Could you check a few things on this model? Use its own coordinates, in mm. Face numbers are marked on the shaded views. A direction names the side the tool comes from. Give positions to 0.01 mm unless a question says otherwise; leave off trailing zeros. Write each loop counter-clockwise with the first axis right and the second up, starting at its lowest first coordinate (ties: lowest second). Pieces come first, ordered by that corner, then holes. Notation, with made-up numbers: M 7.25,59 L 47.25,59 A20 cw 47.25,95 Z; hole C -16.75,42 d11. An arc over 180 degrees is marked long. One line per item, written item: value.
```python
from build123d import *

# Parameters (mm, degrees)
F0_R     = 7.3
F1_DEPTH = 2
F2_R     = 5
F3_DEPTH = 2
F4_SIZE  = 0.5
F5_R     = 2
F6_DEPTH = 4.001


with BuildPart() as f1:
    # F0 (on Top) → F1 (new body)
    with BuildSketch(Plane.XY):
        Circle(F0_R)
    extrude(amount=F1_DEPTH)

    # F2 (on face) → F3 (join)
    with BuildSketch(Plane.XY.offset(2)):
        Circle(F2_R)
    extrude(amount=F3_DEPTH)

    # F4
    f4_edges = [f1.edges().sort_by_distance(p)[0] for p in [
        (-7.3, 0, 0),
    ]]
    chamfer(f4_edges, length=F4_SIZE)

    # F5 (on face) → F6 (cut, through all)
    with BuildSketch(Plane(origin=(0, 0, 0), x_dir=(1, 0, 0), z_dir=(0, 0, -1))):
        Circle(F5_R)
    extrude(amount=-F6_DEPTH, mode=Mode.SUBTRACT)


solid = f1.part
```
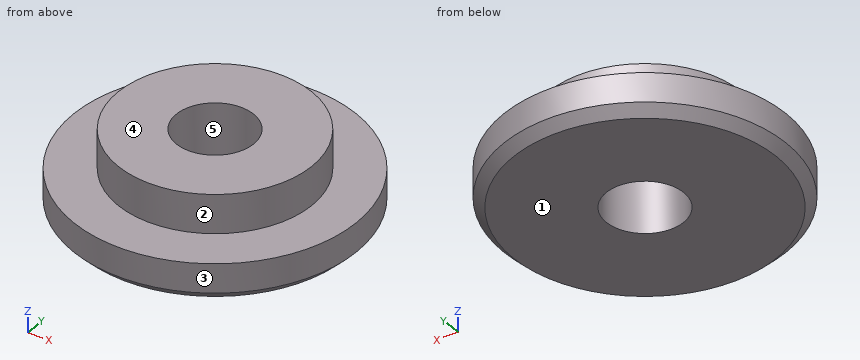
1) On a 3-axis mill with a long thin cutter (end or side, diameter ignored), from which of +Z, -Z, +X, -X, +Y, -Y can I reach the whole of each face in a straight line? I mean the marked faces 1 and 2. Say none if no direction works.
Outcome:
face 1: -Z, +X, -X, +Y, -Y
face 2: +Z
2) Please list where these lines run through material, in increasing order: L1, parallel to Y at x = 0, z = 0.95; L2, parallel to Y at x = 0, z = 2.85; L3, parallel to Z at x = 3.25, y = 5.25. Write a range as from..to.
Outcome:
L1: y = -7.3..-2, 2..7.3
L2: y = -5..-2, 2..5
L3: z = 0..2
3) If we section it at C-C, the plane z = 2.5: Write out the boundary of the cut face in (x, y).
Outcome:
outline: C 0,0 d10; hole C 0,0 d4
4) We'd pull the mould along Y, two halves only. Please class the marked faces 3, 4 and 5: pulls with the +Y half, pulls with the -Y half, needs draft (parallel to the pull), parting line crosses it, or undercut.
Outcome:
face 3: parting line crosses it
face 4: needs draft
face 5: undercut
5) If we section it at A-A, the plane y = 0: Write out the boundary of the cut face in (x, z), then the cut area to 4 significant figures.
Outcome:
outline: M -7.3,0.5 L -6.8,0 L -2,0 L -2,4 L -5,4 L -5,2 L -7.3,2 Z; M 2,0 L 6.8,0 L 7.3,0.5 L 7.3,2 L 5,2 L 5,4 L 2,4 Z
area: 32.95 mm^2
6) I'm going to push a flat-ended pin straight in: pin 1 (5 mm diameter, centred on x = 0, y = 0, fed in from -Z). Where does the tip first touch, or does it pass through?
Outcome:
pin 1: stops at z = 0
